For this review, take the finished solid that the model builds, in its own axes (mm). A direction names the side the tool comes from. Coordinates: 2 decimals unless noted, no trailing zeros. Loops run counter-clockwise (first coordinate to the right, second up) from the corner with the lowest first, then second, coordinate; pieces in that order, holes last. Notation, with made-up numbers: (51, -10) -> (90, -10) arc R24 cw to (90, 16) -> close; hole circle Ø2 at (17, 47.25). An arc over 180 degrees is marked (long way). Use a Markdown table: item, result.
Autodesk Inventor part; units mm, degrees
ref_plane "YZ Plane" through (0, 0, 0) normal (1, 0, 0) x (0, 1, 0)
ref_plane "XZ Plane" through (0, 0, 0) normal (0, 1, 0) x (-1, 0, 0)
ref_plane "XY Plane" through (0, 0, 0) normal (0, 0, 1) x (1, 0, 0)
sketch "Sketch1" plane through (0, 0, 0) normal (0, 0, 1) x (1, 0, 0)
  line L0 (-10, 10) -> (10, 10)
  line L1 (10, 10) -> (10, -10)
  line L2 (10, -10) -> (-10, -10)
  line L3 (-10, -10) -> (-10, 10)
  line L4 (-10, 10) -> (10, -10) construction
  line L5 (10, 10) -> (-10, -10) construction
  point P0 (0, 0)
  dimension "d0" = 20
  dimension "d1" = 20
extrude "Extrusion1" add sketch "Sketch1" along normal blind 2
sketch "Sketch2" plane through (0, 0, 2) normal (0, 0, 1) x (1, 0, 0)
  line L0 (10, 10) -> (-10, 10)
  line L1 (-10, -10) -> (10, -10)
  line L2 (10, 10) -> (8, 10)
  line L3 (8, 10) -> (8, -10)
  line L4 (8, -10) -> (10, -10)
  line L5 (10, -10) -> (10, 10)
  point P0 (0, 0)
  dimension "d4" = 2
extrude "Extrusion2" add sketch "Sketch2" along normal blind 19
sketch "Sketch3" plane through (10, -10, 0) normal (1, 0, 0) x (0, 0, -1)
  circle A0 centre (-11, 10) radius 5
  point P0 (0, 10)
  dimension "d7" = 10
extrude "Extrusion3" cut sketch "Sketch3" against normal up to surface (2 mm away)
properties part number "Holder for Main_Shaft"
(1) Mouldability with a two-part tool opening along Y and no side actions: class faces 1 (the face through (8.2, -10, 5.8)), 2 (the face through (9.01, 1.5, 6.23)), 3 (the face through (9, 0, 21)) as pulls with the +Y half, pulls with the -Y half, needs draft (parallel to the pull), parting line crosses it, or undercut.
Found:
| item | result |
|---|---|
| face 1 | pulls with the -Y half |
| face 2 | undercut |
| face 3 | needs draft |
(2) For pin 1 Ø12 at (y, z) = (3, 14) entering from -X; pin 2 Ø10 at (y, z) = (2, 5.5) entering from -X; pin 3 Ø9 at (x, y) = (-3.5, -2) entering from +Z, all flat-tipped, find the tip position at first contact; note any pin that passes through.
Found:
| item | result |
|---|---|
| pin 1 | stops at x = 8 |
| pin 2 | stops at x = -10 |
| pin 3 | stops at z = 2 |
(3) Take a section at B-B on z = 11. Write out the cut boundary in (x, y).
Found:
| item | result |
|---|---|
| outline | (8, -10) -> (10, -10) -> (10, -5) -> (8, -5) -> close; (8, 5) -> (10, 5) -> (10, 10) -> (8, 10) -> close |
(4) Take a section at D-D on z = 13.5. Write out the cut boundary in (x, y).
Found:
| item | result |
|---|---|
| outline | (8, -10) -> (10, -10) -> (10, -4.33) -> (8, -4.33) -> close; (8, 4.33) -> (10, 4.33) -> (10, 10) -> (8, 10) -> close |
(5) Take a section at C-C on y = 6.5. Write out the cut boundary in (x, z).
Found:
| item | result |
|---|---|
| outline | (-10, 0) -> (10, 0) -> (10, 21) -> (8, 21) -> (8, 2) -> (-10, 2) -> close |
(6) For line 1 along Y through (x, z) = (8.5, 11); line 2 along X through (y, z) = (-7, 17.5); line 3 along Z through (x, y) = (-4, -2.75), list the stretches that pass through material, from the lowest coordinate up.
Found:
| item | result |
|---|---|
| line 1 | y = -10 to -5, 5 to 10 |
| line 2 | x = 8 to 10 |
| line 3 | z = 0 to 2 |
(7) Take a section at A-A on y = 0. Write out the cut boundary in (x, z), plus the area to 3 significant figures.
Found:
| item | result |
|---|---|
| outline | (-10, 0) -> (10, 0) -> (10, 6) -> (8, 6) -> (8, 2) -> (-10, 2) -> close; (8, 16) -> (10, 16) -> (10, 21) -> (8, 21) -> close |
| area | 58.0 mm^2 |
(8) For faces 4 (the face through (0, 0, 0)), 5 (the face through (8, 2, 16)), list the 3-axis set-ups (+Z, -Z, +X, -X, +Y, -Y) from which the entire face can be reached by the end or side of a thin tool; tool diameter is ignored.
Found:
| item | result |
|---|---|
| face 4 | -Z, +X, -X, +Y, -Y |
| face 5 | +Z, -X, +Y, -Y |
